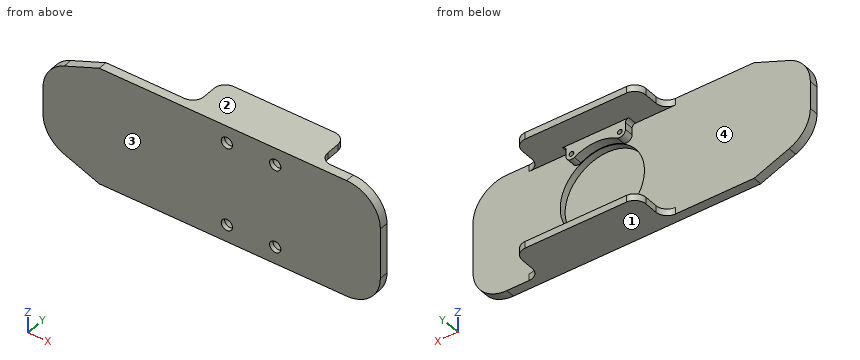
from build123d import *

# Parameters (mm, degrees)
EXTRUDE_1_DEPTH        = 52.5
SKETCH_3_W             = 60
SKETCH_3_H             = 105
CUT_EXTRUDE_1_DEPTH    = 32
SKETCH_4_W             = 54
SKETCH_4_H             = 71
SKETCH_4_R             = 9.5
EXTRUDE_3_DEPTH        = 22.5
SKETCH_4_3_W           = 54
SKETCH_4_3_H           = 71
SKETCH_4_3_R           = 9.5
CUT_EXTRUDE_2_DEPTH    = 14.5
SKETCH_5_R             = 9.5
SKETCH_5_R_2           = 8
EXTRUDE_4_DEPTH        = 2
EXTRUDE_START          = -2
SKETCH_6_R             = 9.5
SKETCH_6_R_2           = 8
EXTRUDE_5_DEPTH        = 2
FILLET_1_R             = 14
FILLET_1_OF_MIRROR_2_R = 14
SKETCH_8_W             = 95
SKETCH_8_H             = 78.931088685
CUT_EXTRUDE_4_DEPTH    = 130
SKETCH_10_W            = 100
SKETCH_10_H            = 93
CUT_EXTRUDE_6_DEPTH    = 32
CUT_EXTRUDE_7_DEPTH    = 73
SKETCH_12_W            = 19.42301832
SKETCH_12_H            = 121.860085881
CUT_EXTRUDE_8_DEPTH    = 73
CUT_EXTRUDE_10_DEPTH   = 150
SKETCH_15_R            = 2.05
SKETCH_15_R_2          = 37.5
CUT_EXTRUDE_11_DEPTH   = 313.725518626
SKETCH_18_W            = 61.222247188
SKETCH_18_H            = 97.808163194
CUT_EXTRUDE_13_DEPTH   = 170
SKETCH_19_R            = 37.5
EXTRUDE_6_DEPTH        = 2
FILLET_2_R             = 30
SKETCH_21_W            = 132.10932858
SKETCH_21_H            = 125.518868867
CUT_EXTRUDE_15_DEPTH   = 149
MM_1_D                 = 10
MM_1_DEPTH             = 4
MM_1_TIP               = 3.004303095
SKETCH_23_W            = 93
SKETCH_23_H            = 32
CUT_EXTRUDE_16_DEPTH   = 149
FILLET_3_R             = 10
EXTRUDE_START_2        = 8
EXTRUDE_8_DEPTH        = 8
CUT_EXTRUDE_START      = -47
SKETCH_27_R            = 2.05
CUT_EXTRUDE_18_DEPTH   = 47
FILLET_4_R             = 3


with BuildPart() as part:
    # 草图1 → 凸台-拉伸1 (new, symmetric)
    with BuildSketch(Plane.XY):
        Polygon((0, 0), (300, 0), (300, 40), (130, 40), (0, 8), align=None)
    extrude(amount=EXTRUDE_1_DEPTH, both=True)

    # 草图3 → 切除-拉伸1 (cut)
    with BuildSketch(Plane(origin=(0, 40, 0), x_dir=(1, 0, 0), z_dir=(0, 1, 0))):
        with Locations((270, 0)):
            Rectangle(SKETCH_3_W, SKETCH_3_H)
    extrude(amount=-CUT_EXTRUDE_1_DEPTH, mode=Mode.SUBTRACT)

    # 草图4 → 凸台-拉伸3 (add, symmetric)
    with BuildSketch(Plane.XY.offset(30)):
        with Locations((273, 43.5)):
            Rectangle(SKETCH_4_W, SKETCH_4_H)
        with Locations(Location((260, 65, 0), (0, 0, 180))):
            Circle(SKETCH_4_R, mode=Mode.SUBTRACT)
    extrude_3 = extrude(amount=EXTRUDE_3_DEPTH, both=True)

    # 草图4<3> → 切除-拉伸2 (cut, symmetric)
    with BuildSketch(Plane.XY.offset(30)):
        with Locations((273, 43.5)):
            Rectangle(SKETCH_4_3_W, SKETCH_4_3_H)
        with Locations(Location((260, 65, 0), (0, 0, 180))):
            Circle(SKETCH_4_3_R, mode=Mode.SUBTRACT)
    cut_extrude_2 = extrude(amount=CUT_EXTRUDE_2_DEPTH, both=True, mode=Mode.SUBTRACT)

    # 草图5 → 凸台-拉伸4 (add)
    with BuildSketch(Plane(origin=(0, 0, 44.5), x_dir=(-1, 0, 0), z_dir=(0, 0, -1))):
        with Locations((-260, 65)):
            Circle(SKETCH_5_R)
        with Locations((-260, 65)):
            Circle(SKETCH_5_R_2, mode=Mode.SUBTRACT)
    extrude_4 = extrude(amount=-EXTRUDE_4_DEPTH)

    # 草图6 → 凸台-拉伸5 (add)
    with BuildSketch(Plane.XY.offset(15.5).offset(EXTRUDE_START)):
        with Locations(Location((260, 65, 0), (0, 0, 180))):
            Circle(SKETCH_6_R)
        with Locations(Location((260, 65, 0), (0, 0, 180))):
            Circle(SKETCH_6_R_2, mode=Mode.SUBTRACT)
    extrude_5 = extrude(amount=EXTRUDE_5_DEPTH)

    # 圆角1
    fillet_1_edges = [part.edges().sort_by_distance(p)[0] for p in [
        (246, 79, 48.5),
        (246, 79, 11.5),
    ]]
    fillet(fillet_1_edges, radius=FILLET_1_R)

    # 镜向2: 凸台-拉伸3, 切除-拉伸2, 凸台-拉伸4, 凸台-拉伸5 across plane
    add(extrude_3.mirror(Plane.XY))
    add(cut_extrude_2.mirror(Plane.XY), mode=Mode.SUBTRACT)
    add(extrude_4.mirror(Plane.XY))
    add(extrude_5.mirror(Plane.XY))

    # 圆角1 of 镜向2
    fillet_1_of_mirror_2_edges = [part.edges().sort_by_distance(p)[0] for p in [
        (246, 79, -48.5),
        (246, 79, -11.5),
    ]]
    fillet(fillet_1_of_mirror_2_edges, radius=FILLET_1_OF_MIRROR_2_R)

    # 草图8 → 切除-拉伸4 (cut)
    with BuildSketch(Plane.ZY):
        with Locations((0, 47.465544343)):
            Rectangle(SKETCH_8_W, SKETCH_8_H)
    extrude(amount=-CUT_EXTRUDE_4_DEPTH, mode=Mode.SUBTRACT)

    # 草图10 → 切除-拉伸6 (cut)
    with BuildSketch(Plane(origin=(0, 40, 0), x_dir=(1, 0, 0), z_dir=(0, 1, 0))):
        with Locations((185, 0)):
            Rectangle(SKETCH_10_W, SKETCH_10_H)
    extrude(amount=-CUT_EXTRUDE_6_DEPTH, mode=Mode.SUBTRACT)

    # 草图11 → 切除-拉伸7 (cut)
    with BuildSketch(Plane.XZ):
        Polygon((-14.613233699, 52.5), (50.030946001, 52.5), (0, 32.5), (0, -32.5), (50, -52.5), (-14.613233699, -52.5), align=None)
    extrude(amount=-CUT_EXTRUDE_7_DEPTH, mode=Mode.SUBTRACT)

    # 草图12 → 切除-拉伸8 (cut)
    with BuildSketch(Plane(origin=(0, 8, 0), x_dir=(1, 0, 0), z_dir=(0, 1, 0))):
        with Locations((40.28849084, -8.430042941)):
            Rectangle(SKETCH_12_W, SKETCH_12_H)
    extrude(amount=CUT_EXTRUDE_8_DEPTH, mode=Mode.SUBTRACT)

    # 草图14 → 切除-拉伸10 (cut, symmetric)
    with BuildSketch(Plane.XY.offset(52.5)):
        with BuildLine():
            Line((275.075376069, 79), (318.037843951, 79))
            Line((318.037843951, 79), (300, 8))
            ThreePointArc((300, 8), (292.070381124, 45.091206629), (275.075376069, 79))
        make_face()
    extrude(amount=CUT_EXTRUDE_10_DEPTH, both=True, mode=Mode.SUBTRACT)

    # 草图15 → 切除-拉伸11 (cut, through all)
    with BuildSketch(Plane(origin=(0, 8, 0), x_dir=(1, 0, 0), z_dir=(0, 1, 0))):
        with Locations(Location((163.5, -37.239092363, 0), (0, 0, 180))):
            Circle(SKETCH_15_R)
        with Locations((163.5, 37.239092363)):
            Circle(SKETCH_15_R)
        with Locations(Location((206.5, 37.239092363, 0), (0, 0, 180))):
            Circle(SKETCH_15_R)
        with Locations((206.5, -37.239092363)):
            Circle(SKETCH_15_R)
        with Locations(Location((185, 0, 0), (0, 0, 180))):
            Circle(SKETCH_15_R_2)
    extrude(amount=-CUT_EXTRUDE_11_DEPTH, mode=Mode.SUBTRACT)

    # 草图18 → 切除-拉伸13 (cut)
    with BuildSketch(Plane.XY.offset(52.5)):
        with Locations((276.611123594, 56.904081597)):
            Rectangle(SKETCH_18_W, SKETCH_18_H)
    extrude(amount=-CUT_EXTRUDE_13_DEPTH, mode=Mode.SUBTRACT)

    # 草图19 → 凸台-拉伸6 (add)
    with BuildSketch(Plane.XZ.offset(EXTRUDE_START)):
        with Locations(Location((185, 0, 0), (0, 0, 180))):
            Circle(SKETCH_19_R)
    extrude(amount=EXTRUDE_6_DEPTH)

    # 圆角2
    fillet_2_edges = [part.edges().sort_by_distance(p)[0] for p in [
        (300, 4, 52.5),
        (0, 4, 32.5),
        (0, 4, -32.5),
        (300, 4, -52.5),
    ]]
    fillet(fillet_2_edges, radius=FILLET_2_R)

    # 草图21 → 切除-拉伸15 (cut)
    with BuildSketch(Plane(origin=(0, 8, 0), x_dir=(1, 0, 0), z_dir=(0, 1, 0))):
        with Locations((63.94533571, -10.259434434)):
            Rectangle(SKETCH_21_W, SKETCH_21_H)
    extrude(amount=CUT_EXTRUDE_15_DEPTH, mode=Mode.SUBTRACT)

    # 大小mm 暗销孔1
    with Locations(Plane(origin=(163.5, 0, 37.239092363), x_dir=(0, 0, -1), z_dir=(0, -1, 0))):
        with Locations((0, 0), (0, 43), (74.478184726, 43), (74.478184726, 0)):
            Hole(MM_1_D / 2, depth=MM_1_DEPTH)
            with Locations((0, 0, -(MM_1_DEPTH + MM_1_TIP / 2))):  # 118° drill point
                Cone(0, MM_1_D / 2, MM_1_TIP, mode=Mode.SUBTRACT)

    # 草图23 → 切除-拉伸16 (cut)
    with BuildSketch(Plane.ZY.offset(-130)):
        with Locations((0, 24)):
            Rectangle(SKETCH_23_W, SKETCH_23_H)
    extrude(amount=-CUT_EXTRUDE_16_DEPTH, mode=Mode.SUBTRACT)

    # 圆角3
    fillet_3_edges = [part.edges().sort_by_distance(p)[0] for p in [
        (130, 8, -49.5),
        (240, 40, -49.5),
        (240, 8, 49.5),
        (130, 8, 49.5),
        (130, 40, -49.5),
        (240, 8, -49.5),
        (240, 40, 49.5),
        (130, 40, 49.5),
    ]]
    fillet(fillet_3_edges, radius=FILLET_3_R)

    # 草图26 → 凸台-拉伸8 (add)
    with BuildSketch(Plane(origin=(0, 8, 0), x_dir=(1, 0, 0), z_dir=(0, 1, 0)).offset(EXTRUDE_START_2)):
        with BuildLine():
            Line((158.5, 46.5), (158.5, 37.239092363))
            ThreePointArc((158.5, 37.239092363), (161, 32.908965344), (166, 32.908965344))
            ThreePointArc((166, 32.908965344), (185, 38), (204, 32.908965344))
            ThreePointArc((204, 32.908965344), (209, 32.908965344), (211.5, 37.239092363))
            Line((211.5, 37.239092363), (211.5, 46.5))
            Line((211.5, 46.5), (211.5, 50.5))
            Line((211.5, 50.5), (158.5, 50.5))
            Line((158.5, 50.5), (158.5, 46.5))
        make_face()
        with BuildLine():
            Line((211.5, -46.495333446), (211.5, -37.234425809))
            ThreePointArc((211.5, -37.234425809), (209, -32.90429879), (204, -32.90429879))
            ThreePointArc((204, -32.90429879), (185, -37.995333446), (166, -32.90429879))
            ThreePointArc((166, -32.90429879), (161, -32.90429879), (158.5, -37.234425809))
            Line((158.5, -37.234425809), (158.5, -46.495333446))
            Line((158.5, -46.495333446), (158.5, -50.495333446))
            Line((158.5, -50.495333446), (211.5, -50.495333446))
            Line((211.5, -50.495333446), (211.5, -46.495333446))
        make_face()
    extrude(amount=-EXTRUDE_8_DEPTH)

    # 草图27 → 切除-拉伸18 (cut)
    with BuildSketch(Plane.XZ.offset(CUT_EXTRUDE_START)):
        with Locations(Location((206.5, -37.239092363, 0), (0, 0, 270))):
            Circle(SKETCH_27_R)
        with Locations(Location((163.5, -37.239092363, 0), (0, 0, 270))):
            Circle(SKETCH_27_R)
        with Locations(Location((163.5, 37.239092363, 0), (0, 0, 90))):
            Circle(SKETCH_27_R)
        with Locations(Location((206.5, 37.239092363, 0), (0, 0, 90))):
            Circle(SKETCH_27_R)
    extrude(amount=CUT_EXTRUDE_18_DEPTH, mode=Mode.SUBTRACT)

    # 圆角4
    fillet_4_edges = [part.edges().sort_by_distance(p)[0] for p in [
        (211.5, 12, -46.5),
        (158.5, 12, -46.5),
        (211.5, 12, 46.5),
        (158.5, 12, 46.5),
    ]]
    fillet(fillet_4_edges, radius=FILLET_4_R)


solid = part.part
The model under review builds one solid part; all positions refer to its coordinate system, in mm. Face numbers are marked on the shaded views. Give positions to 0.01 mm unless a question says otherwise; leave off trailing zeros. Loops run counter-clockwise (first coordinate to the right, second up) from the corner with the lowest first, then second, coordinate; pieces in that order, holes last. Notation, with made-up numbers: (44, 36) -> (64, 36) arc R26 ccw to (64, 62) -> close; hole circle Ø9 at (26, -15.75). An arc over 180 degrees is marked (long way). Put each result on its own line as item: value. Start each with the question number.
1. Wall thickness on probe 1 along X at (y, z) = (3.5, 40); probe 2 along Z at (x, y) = (163, 3); probe 3 along Z at (x, y) = (206.5, 6.3): over which ranges is each line inside the solid? List them lowest first.
2. We need section D-D on x = 116.5. State the section outline as (y, z) points.
3. Mouldability with a two-part tool opening along Z and no side actions: class the marked faces 1, 2, 3 and 4 as released by +Z, released by -Z, zero draft, split by the parting line, or undercut.
4. We need section A-A on z = 0. State the section outline as (x, y) points.
5. We need section C-C on z = 27. State the section outline as (x, y) points.
6. We need section B-B on x = 185. State the section outline as (y, z) points, then the cut area to 3 significant figures.
7. Clearance check with flat-ended pins moving along their axes: P1, Ø1.9, axis at y = 11, z = 41.5, coming from the +X side; P2, Ø4.5, axis at x = 163.5, z = 37.24, coming from the -Y side; P3, Ø1.5, axis at y = 5, z = -37.5, coming from the +X side. State where each tip first meets the part, or that it passes through.
Determined:
1. probe 1: 18.76 to 159.33, 167.67 to 202.33, 210.67 to 294.37
1. probe 2: -52.5 to -42.21, -32.26 to -30.37, 30.37 to 32.26, 42.21 to 52.5
1. probe 3: -52.5 to -39.29, -35.19 to -30.72, 30.72 to 35.19, 39.29 to 52.5
2. outline: (0, -52.5) -> (8, -52.5) -> (8, 52.5) -> (0, 52.5) -> close
3. face 1: released by -Z
3. face 2: released by +Z
3. face 3: zero draft
3. face 4: undercut
4. outline: (0, 0) -> (300, 0) -> (300, 8) -> (222.5, 8) -> (222.5, 2) -> (147.5, 2) -> (147.5, 8) -> (0, 8) -> close
5. outline: (3.91, 0) -> (299.66, 0) -> (299.66, 8) -> (211.02, 8) -> (211.02, 2) -> (158.98, 2) -> (158.98, 8) -> (3.91, 8) -> close
6. outline: (0, -52.5) -> (40, -52.5) -> (40, -46.5) -> (16, -46.5) -> (16, -38) -> (8, -38) -> (8, -37.5) -> (2, -37.5) -> (2, 37.5) -> (8, 37.5) -> (8, 38) -> (16, 38) -> (16, 46.5) -> (40, 46.5) -> (40, 52.5) -> (0, 52.5) -> close
6. area: 910 mm^2
7. P1: x = 211.5
7. P2: y = 5.65
7. P3: x = 296.4
